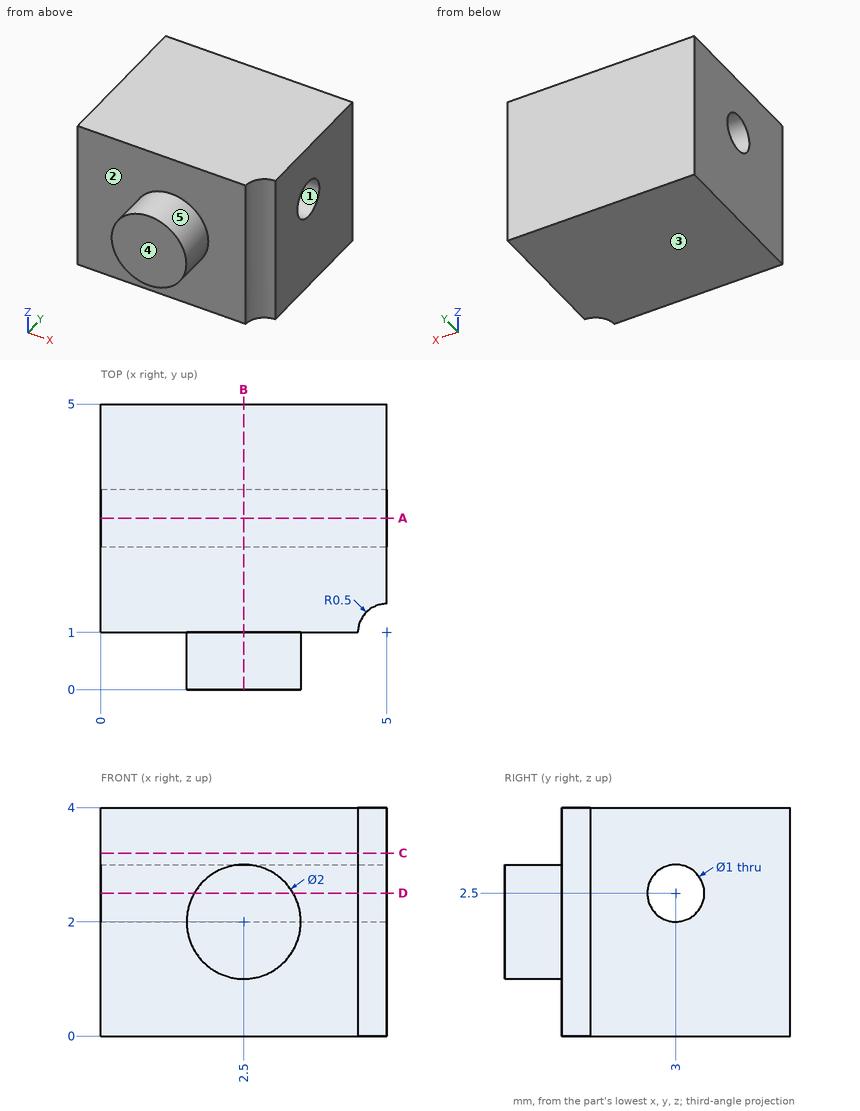
For this review, use the dimensioned drawing (mm, ordinates from the lowest corner) and the shaded views. A direction names the side the tool comes from. Give positions to 0.01 mm unless a question says otherwise; leave off trailing zeros. Order: outer loops, then holes, each group sorted by start corner. A loop starts at its lowest first (then second) coordinate and runs counter-clockwise, first axis right, second up.
1) Take a section at C-C (z = 3.2). Give the boundary of the cut face in (x, y).
2) Wall thickness on line 1 (Z direction, x = 1, y = 3); line 2 (Y direction, x = 2, z = 1.1); line 3 (Y direction, x = 2.2, z = 2.45): over which ranges is each line inside the solid? List them lowest first.
3) For the marked faces 4 and 5, list the 3-axis set-ups (+Z, -Z, +X, -X, +Y, -Y) from which the entire face can be reached by the end or side of a thin tool; tool diameter is ignored.
4) Take a section at A-A (y = 3). Give the boundary of the cut face in (x, z), then the cut area to 3 significant figures.
5) Take a section at B-B (x = 2.5). Give the boundary of the cut face in (y, z), then the cut area to 3 significant figures.
6) Take a section at D-D (z = 2.5). Give the boundary of the cut face in (x, y).
7) The part is to be moulded in two halves that separate along Z. For the marked faces 1, 2 and 3, say which applies: released by +Z, released by -Z, zero draft, split by the parting line, or undercut.
Derived:
1. outline: (0, 1) - (4.5, 1) arc R0.5 cw to (5, 1.5) - (5, 5) - (0, 5) - close
2. line 1: z = 0 to 2, 3 to 4
2. line 2: y = 1 to 5
2. line 3: y = 0 to 2.5, 3.5 to 5
3. face 4: +Z, -Z, +X, -X, -Y
3. face 5: -Y
4. outline: (0, 0) - (5, 0) - (5, 2) - (0, 2) - close; (0, 3) - (5, 3) - (5, 4) - (0, 4) - close
4. area: 15.0 mm2
5. outline: (0, 1) - (1, 1) - (1, 0) - (5, 0) - (5, 4) - (1, 4) - (1, 3) - (0, 3) - close; hole circle Ø1 at (3, 2.5)
5. area: 17.2 mm2
6. outline: (0, 1) - (1.63, 1) - (1.63, 0) - (3.37, 0) - (3.37, 1) - (4.5, 1) arc R0.5 cw to (5, 1.5) - (5, 2.5) - (0, 2.5) - close; (0, 3.5) - (5, 3.5) - (5, 5) - (0, 5) - close
7. face 1: undercut
7. face 2: zero draft
7. face 3: released by -Z
